```python
from build123d import *

# Parameters (mm, degrees)
PAD_DEPTH               = 5
SKETCH002_R             = 1.15
POCKET_DEPTH            = 5.001
POCKET_DEPTH_BACK       = 0.001
BODY001_PLACEMENT_ANGLE = 5


with BuildPart() as part:
    # Sketch → Pad (new body)
    with BuildSketch(Plane.XY):
        with BuildLine():
            ThreePointArc((-4, 0), (0, -4), (4, 0))
            ThreePointArc((4, 0), (3.532704, 1.876167), (2.239999, 3.313971))
            ThreePointArc((1.995291, 6.433002), (1.366125, 4.814525), (2.239999, 3.313971))
            ThreePointArc((8, 8.800007), (4.772802, 8.186896), (1.995291, 6.433002))
            ThreePointArc((26.730076, 7.183219), (17.399864, 8.39506), (8, 8.800007))
            ThreePointArc((28.315082, 5.745575), (27.73102, 6.694204), (26.730076, 7.183219))
            ThreePointArc((28.315082, 5.745575), (30.204969, 3.966171), (32.655215, 4.823051))
            ThreePointArc((34.687932, 5.491725), (33.574624, 5.452108), (32.655215, 4.823051))
            ThreePointArc((85.286771, -23.213222), (61.932163, -5.432587), (34.687932, 5.491725))
            ThreePointArc((85.286771, -23.213222), (87.549513, -23.213222), (87.549513, -20.95048))
            ThreePointArc((87.549513, -20.95048), (51.051886, 3.436454), (8, 12.000007))
            ThreePointArc((8, 12.000007), (-0.485282, 8.485284), (-4, 0))
        make_face()
    extrude(amount=-PAD_DEPTH)

    # Sketch002 → Pocket (cut, two sides)
    with BuildSketch(Plane.XY) as pocket_sk:
        with Locations((30.724748, 6.411535)):
            Circle(SKETCH002_R)
    extrude(amount=-POCKET_DEPTH, mode=Mode.SUBTRACT)
    extrude(pocket_sk.sketch, amount=POCKET_DEPTH_BACK, mode=Mode.SUBTRACT)

    # Sketch003 → Groove (revolve, cut)
    with BuildSketch(Plane.XZ):
        Polygon((0, 0), (3.9, 0), (2.65, -1.25), (2.65, -3.75), (3.9, -5), (0, -5), align=None)
    revolve(axis=Axis((0, 0, 0), (0, 0, 1)), mode=Mode.SUBTRACT)


with BuildPart() as part_1:
    # Body001 placement: moved
    add(part.part.moved(Location((0, 0, -6))).rotate(Axis((0, 0, -6), (0, 0, -1)), BODY001_PLACEMENT_ANGLE))


solid = part_1.part
```
Work out the finished part from the listing and answer in its coordinate system (mm). A direction names the side the tool comes from. Give positions to 0.01 mm unless a question says otherwise; leave off trailing zeros. Loops run counter-clockwise (first coordinate to the right, second up) from the corner with the lowest first, then second, coordinate; pieces in that order, holes last. Notation, with made-up numbers: (-5, 3.5) - (38, 3.5) arc R18 ccw to (38, 34.5) - close; hole circle Ø4 at (34, 63.25). An arc over 180 degrees is marked (long way). Use CSV: the item, a comma, the result in double quotes. Start each with the question number.
(1) Determine the mould class of faces 4 (the face through (42, 0, -11)), 5 (the face through (33.9, 2.5, -8.5)), 6 (the face through (-0.115, 2.648, -8.518)) for opening direction Y: released by +Y, released by -Y, zero draft, split by the parting line, or undercut.
(2) Find section A-A, the plane x = 0. Determine the outline of the cut face in (y, z), plus the area to 3 significant figures.
(3) Find the intervals of material crossed by L1, parallel to X at y = 0, z = -8.5; L2, parallel to X at y = 3, z = -8.55; L3, parallel to Y at x = 0, z = -8.9, in increasing order.
(4) Find section C-C, the plane x = 70. Determine the outline of the cut face in (y, z).
(5) Find section B-B, the plane z = -8.95. Determine the outline of the cut face in (x, y).
(6) Find section D-D, the plane y = -20.5. Determine the outline of the cut face in (x, z).
(7) A tool of negligible diameter and unlimited length cuts with its end or side. For faces 1 (the face through (42, 0, -6)), 2 (the face through (61.562, -11.044, -8.465)), 3 (the face through (1.78, 4.7, -8.46)), from which of +Z, -Z, +X, -X, +Y, -Y can it reach the whole face along a straight path? Write none if from no direction.
(8) Each of these flat-tipped pins is pushed along its axis until it touches: pin 1 (3 mm diameter, centred on x = 9.5, y = 6, fed in from +Z); pin 2 (1 mm diameter, centred on y = -6.5, z = -8.5, fed in from +X); pin 3 (2 mm diameter, centred on y = -23, z = -6.5, fed in from -X); pin 4 (7 mm diameter, centred on x = 0, y = 0, fed in from +Z). Where does it stop, or does it pass through?
Results found:
1,face 4,"zero draft"
1,face 5,"released by -Y"
1,face 6,"undercut"
2,outline,"(-4, -11) - (-3.9, -11) - (-2.65, -9.75) - (-2.65, -7.25) - (-3.9, -6) - (-4, -6) - close; (2.65, -9.75) - (3.9, -11) - (8.27, -11) - (8.27, -6) - (3.9, -6) - (2.65, -7.25) - close"
2,area,"31.7 mm^2"
3,L1,"-4 to -2.65, 2.65 to 4, 41.43 to 49.14"
3,L2,"-3.45 to 2.65, 28.77 to 30.26, 32.07 to 42.55"
3,L3,"-4 to -2.65, 2.65 to 8.27"
4,outline,"(-17.54, -11) - (-13.38, -11) - (-13.38, -6) - (-17.54, -6) - close"
5,outline,"(-3.98, 0.35) arc R4 ccw (long way) to (2.52, 3.11) arc R2 cw to (2.55, 6.23) arc R8.8 cw to (8.74, 8.07) arc R109.3 cw to (27.25, 4.83) arc R2 cw to (28.71, 3.26) arc R2.5 ccw to (32.95, 1.96) arc R2 cw to (35.03, 2.45) arc R109.3 cw to (82.94, -30.56) arc R1.6 ccw to (85.39, -28.5) arc R112.5 ccw to (9.02, 11.26) arc R12 ccw to start; hole circle Ø5.3 at (0, 0); hole circle Ø2.3 at (31.17, 3.71)"
6,outline,"(73.35, -11) - (77.99, -11) - (77.99, -6) - (73.35, -6) - close"
7,face 1,"+Z, +X, -X, +Y, -Y"
7,face 2,"+Z, -Z, -Y"
7,face 3,"+Z, -Z"
8,pin 1,"through"
8,pin 2,"x = 61.3"
8,pin 3,"x = 74.94"
8,pin 4,"z = -6.4"
